```python
from build123d import *

# Parameters (mm, degrees)
SKETCH_W      = 140
SKETCH_H      = 200
PAD_DEPTH     = 30
FILLET_R      = 8
THICKNESS_T   = -2
SKETCH001_W   = 2
SKETCH001_H   = 196
SKETCH001_W_2 = 43
SKETCH001_H_2 = 2.053146
PAD001_DEPTH  = 28
SKETCH002_W   = 2
SKETCH002_H   = 196
SKETCH002_W_2 = 36.08274
SKETCH002_H_2 = 2.002022
SKETCH002_H_3 = 2.030933
SKETCH002_H_4 = 2.030928
SKETCH002_H_5 = 1.901375
SKETCH002_W_3 = 53.704103
SKETCH002_H_6 = 1.896915
SKETCH002_W_4 = 53
SKETCH002_H_7 = 2.073647
SKETCH002_W_5 = 52.91726
SKETCH002_H_8 = 1.89692
PAD002_DEPTH  = 10
PAD003_DEPTH  = 28
SKETCH003_W   = 43
SKETCH003_H   = 2
PAD004_DEPTH  = 30


with BuildPart() as part:
    # Sketch → Pad (new body)
    with BuildSketch(Plane.XY):
        with Locations((11.803558, 17.899191)):
            Rectangle(SKETCH_W, SKETCH_H)
    extrude(amount=PAD_DEPTH)

    # Fillet
    fillet_edges = [part.edges().sort_by_distance(p)[0] for p in [
        (-58.196442, -82.100809, 15),
        (81.803558, -82.100809, 15),
        (81.803558, 117.899191, 15),
        (-58.196442, 117.899191, 15),
    ]]
    fillet(fillet_edges, radius=FILLET_R)

    # Thickness
    thickness_openings = [part.faces().sort_by_distance(p)[0] for p in [
        (11.803558, 17.899191, 30),
    ]]
    offset(amount=THICKNESS_T, openings=thickness_openings)

    # Sketch001 (on Face10 of Thickness) → Pad001 (join)
    with BuildSketch(Plane.XY.offset(30)):
        with Locations((-12.196442, 17.899191)):
            Rectangle(SKETCH001_W, SKETCH001_H)
        with Locations((-34.696442, 70.620445)):
            Rectangle(SKETCH001_W_2, SKETCH001_H_2)
    extrude(amount=-PAD001_DEPTH)

    # Sketch002 (on Face23 of Pad001) → Pad002 (join)
    with BuildSketch(Plane.XY.offset(2)):
        with Locations((25.886298, 17.899191)):
            Rectangle(SKETCH002_W, SKETCH002_H)
        with Locations((6.844928, 70.562603)):
            Rectangle(SKETCH002_W_2, SKETCH002_H_2)
        with Locations((6.844928, 29.084188)):
            Rectangle(SKETCH002_W_2, SKETCH002_H_3)
        with Locations((6.844928, -12.045896)):
            Rectangle(SKETCH002_W_2, SKETCH002_H_4)
        with Locations((6.844928, -47.510318)):
            Rectangle(SKETCH002_W_2, SKETCH002_H_5)
        with Locations((53.738349, 49.849649)):
            Rectangle(SKETCH002_W_3, SKETCH002_H_6)
        with Locations((53.386298, 16.862367)):
            Rectangle(SKETCH002_W_4, SKETCH002_H_7)
        with Locations((53.344928, -26.393629)):
            Rectangle(SKETCH002_W_5, SKETCH002_H_8)
    extrude(amount=PAD002_DEPTH)

    # Sketch002 (on Face23 of Pad001) → Pad003 (join)
    with BuildSketch(Plane.XY.offset(2)):
        with Locations((25.886298, 17.899191)):
            Rectangle(SKETCH002_W, SKETCH002_H)
        with Locations((6.844928, 70.562603)):
            Rectangle(SKETCH002_W_2, SKETCH002_H_2)
        with Locations((6.844928, 29.084188)):
            Rectangle(SKETCH002_W_2, SKETCH002_H_3)
        with Locations((6.844928, -12.045896)):
            Rectangle(SKETCH002_W_2, SKETCH002_H_4)
        with Locations((6.844928, -47.510318)):
            Rectangle(SKETCH002_W_2, SKETCH002_H_5)
        with Locations((53.738349, 49.849649)):
            Rectangle(SKETCH002_W_3, SKETCH002_H_6)
        with Locations((53.386298, 16.862367)):
            Rectangle(SKETCH002_W_4, SKETCH002_H_7)
        with Locations((53.344928, -26.393629)):
            Rectangle(SKETCH002_W_5, SKETCH002_H_8)
    extrude(amount=PAD003_DEPTH)

    # Sketch003 → Pad004 (join)
    with BuildSketch(Plane.XY):
        with Locations((-34.696442, 29.20466)):
            Rectangle(SKETCH003_W, SKETCH003_H)
        with Locations((-34.696442, -12.11418)):
            Rectangle(SKETCH003_W, SKETCH003_H)
    extrude(amount=PAD004_DEPTH)


solid = part.part
```
CAD build for the part. Positions are in the model's coordinates, mm. A direction names the side the tool comes from. Round coordinates to 2 decimals unless told otherwise and drop trailing zeros. Write each loop counter-clockwise with the first axis right and the second up, starting at its lowest first coordinate (ties: lowest second). Pieces come first, ordered by that corner, then holes. Notation, with made-up numbers: (42, 87.25) -> (62, 87.25) arc R15 ccw to (62, 100.25) -> close; hole circle Ø10 at (-4, -7). An arc over 180 degrees is marked (long way). Answer in a Markdown table with one row per item. Add a question column.
Item 1: Drop a flat-ended pin along its axis: pin 1 Ø12 at (x, y) = (60.5, 68) entering from +Z. Give the stop position or say it passes through.
Item 2: Which spindle directions (+Z, -Z, +X, -X, +Y, -Y) get a long thin tool onto all of the face, cutting with end or side? Do faces 4 (the face through (7, -48.461, 16)), 5 (the face through (-55.92, 115.49, 15.21)). Say none if no direction does.
Item 3: Saw through at C-C, the plane y = 82.5. Write the cut outline in (x, z), then the cut area to 3 significant figures.
Item 4: Saw through at B-B, the plane z = 6.75. Count the separate pieces of the cut face and the enclosed holes in it, then the cut area to 3 significant figures.
Item 5: Mould opens along X. For faces 1 (the face through (79.522, 115.494, 15.21)), 2 (the face through (-56.196, 8, 16)), 3 (the face through (11, -82.101, 15)) say: pulls with the +X half, pulls with the -X half, needs draft (parallel to the pull), parting line crosses it, or undercut.
Item 6: Drill centre lines: line 1 (Y direction, x = -8.5, z = 12); line 2 (Y direction, x = 28, z = 8); line 3 (X direction, y = 51.5, z = 19). Where is each one in solid material? Low to high. Write a range as from..to.
Item 7: Saw through at D-D, the plane x = -43. Write the cut outline in (y, z), then the cut area to 3 significant figures.
Item 8: Saw through at A-A, the plane x = 8. Write the cut outline in (y, z).
Findings below:
| question | item | result |
|---|---|---|
| 1 | pin 1 | stops at z = 2 |
| 2 | face 4 | +Z |
| 2 | face 5 | +Z, -Z, -X, +Y |
| 3 | outline | (-58.2, 0) -> (81.8, 0) -> (81.8, 30) -> (79.8, 30) -> (79.8, 2) -> (26.89, 2) -> (26.89, 30) -> (24.89, 30) -> (24.89, 2) -> (-11.2, 2) -> (-11.2, 30) -> (-13.2, 30) -> (-13.2, 2) -> (-56.2, 2) -> (-56.2, 30) -> (-58.2, 30) -> close |
| 3 | area | 504 mm^2 |
| 4 | separate pieces | 1 |
| 4 | enclosed holes | 13 |
| 4 | area | 2,960 mm^2 |
| 5 | face 1 | pulls with the +X half |
| 5 | face 2 | undercut |
| 5 | face 3 | needs draft |
| 6 | line 1 | y = -82.1..-80.1, -48.46..-46.56, -13.06..-11.03, 28.07..30.1, 69.56..71.56, 115.9..117.9 |
| 6 | line 2 | y = -82.1..-80.1, -27.34..-25.45, 15.83..17.9, 48.9..50.8, 115.9..117.9 |
| 6 | line 3 | x = -58.2..-56.2, -13.2..-11.2, 24.89..26.89, 79.8..81.8 |
| 7 | outline | (-82.1, 0) -> (117.9, 0) -> (117.9, 30) -> (115.9, 30) -> (115.9, 2) -> (71.65, 2) -> (71.65, 30) -> (69.59, 30) -> (69.59, 2) -> (30.2, 2) -> (30.2, 30) -> (28.2, 30) -> (28.2, 2) -> (-11.11, 2) -> (-11.11, 30) -> (-13.11, 30) -> (-13.11, 2) -> (-80.1, 2) -> (-80.1, 30) -> (-82.1, 30) -> close |
| 7 | area | 681 mm^2 |
| 8 | outline | (-82.1, 0) -> (117.9, 0) -> (117.9, 30) -> (115.9, 30) -> (115.9, 2) -> (71.56, 2) -> (71.56, 30) -> (69.56, 30) -> (69.56, 2) -> (30.1, 2) -> (30.1, 30) -> (28.07, 30) -> (28.07, 2) -> (-11.03, 2) -> (-11.03, 30) -> (-13.06, 30) -> (-13.06, 2) -> (-46.56, 2) -> (-46.56, 30) -> (-48.46, 30) -> (-48.46, 2) -> (-80.1, 2) -> (-80.1, 30) -> (-82.1, 30) -> close |
